Study the drawing (mm; zero at the part's minimum x, y, z) and answer. A direction names the side the tool comes from. Coordinates: 2 decimals unless noted, no trailing zeros. Loops run counter-clockwise (first coordinate to the right, second up) from the corner with the lowest first, then second, coordinate; pieces in that order, holes last. Notation, with made-up numbers: (-10.5, 16) -> (23.5, 16) arc R20 ccw to (23.5, 33) -> close; hole circle Ø1 at (78.5, -12). An arc over 180 degrees is marked (long way). Answer in a Markdown table with one row per item.
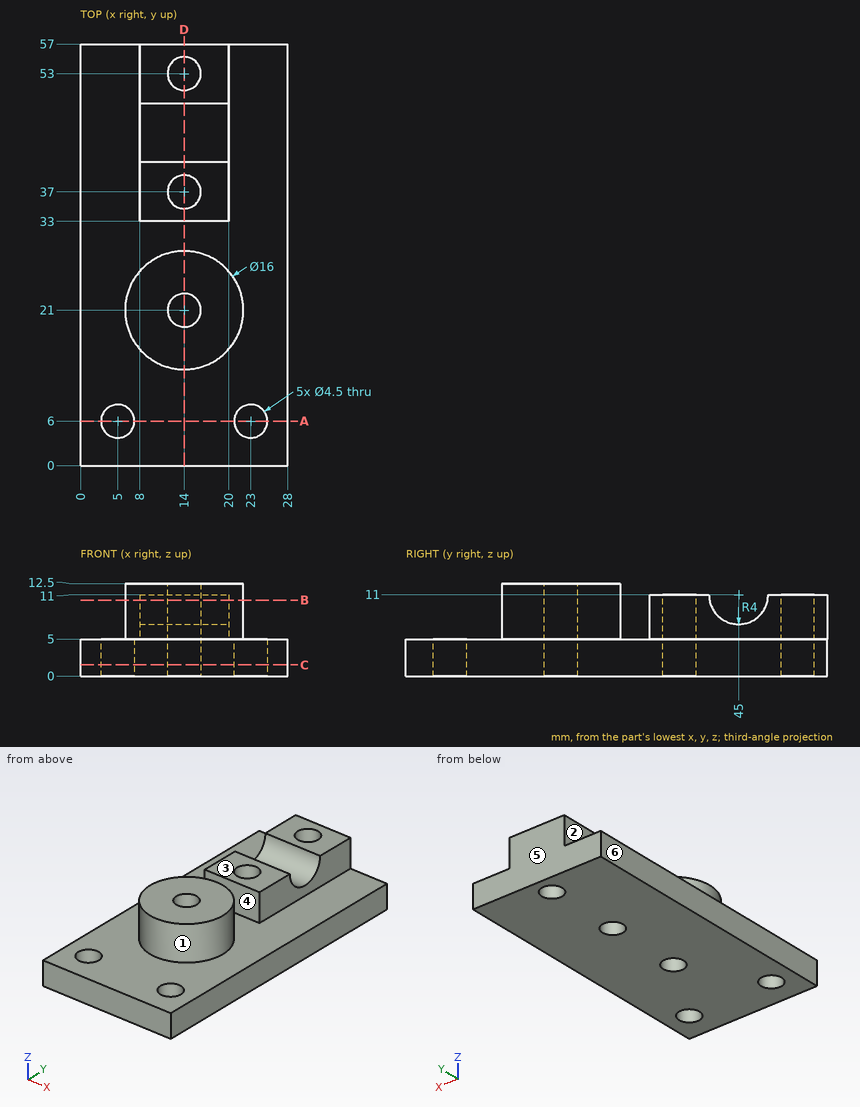
1. Given pin 1 Ø2.5 at (x, y) = (11.5, 38.5) entering from +Z; pin 2 Ø3 at (y, z) = (36, 8.5) entering from -X; pin 3 Ø1 at (y, z) = (46.5, 10.5) entering from -X; pin 4 Ø1.5 at (y, z) = (21.5, 7.5) entering from +X, each flat-ended and moving along its own axis, determine where each tip first touches the part or whether it passes through.
A:
| item | result |
|---|---|
| pin 1 | stops at z = 11 |
| pin 2 | stops at x = 8 |
| pin 3 | passes through |
| pin 4 | stops at x = 22 |
2. The mould has two halves that part along Y. Classify the marked faces 4, 5 and 6: pulls with the +Y half, pulls with the -Y half, needs draft (parallel to the pull), parting line crosses it, or undercut.
A:
| item | result |
|---|---|
| face 4 | undercut |
| face 5 | pulls with the +Y half |
| face 6 | needs draft |
3. A tool of negligible diameter and unlimited length cuts with its end or side. For the marked faces 1, 2 and 3, from which of +Z, -Z, +X, -X, +Y, -Y can it reach the whole face along a straight path? Write none if from no direction.
A:
| item | result |
|---|---|
| face 1 | +Z |
| face 2 | +Z, -X, +Y |
| face 3 | +Z, +X, -X, +Y |
4. A cutting plane is placed at A-A on y = 6. Give the vertices of the cut face in (x, z).
A:
| item | result |
|---|---|
| outline | (0, 0) -> (2.75, 0) -> (2.75, 5) -> (0, 5) -> close; (7.25, 0) -> (20.75, 0) -> (20.75, 5) -> (7.25, 5) -> close; (25.25, 0) -> (28, 0) -> (28, 5) -> (25.25, 5) -> close |
5. Find the intervals of material crossed by probe 1 along Y at (x, z) = (14, 8); probe 2 along Y at (x, z) = (16, 10.5); probe 3 along Y at (x, z) = (14, 6.5), in increasing order.
A:
| item | result |
|---|---|
| probe 1 | y = 13 to 18.75, 23.25 to 29, 33 to 34.75, 39.25 to 42.35, 47.65 to 50.75, 55.25 to 57 |
| probe 2 | y = 13.25 to 19.97, 22.03 to 28.75, 33 to 35.97, 38.03 to 41.03, 48.97 to 51.97, 54.03 to 57 |
| probe 3 | y = 13 to 18.75, 23.25 to 29, 33 to 34.75, 39.25 to 50.75, 55.25 to 57 |
6. A cutting plane is placed at C-C on z = 1.5. Give the vertices of the cut face in (x, y).
A:
| item | result |
|---|---|
| outline | (0, 0) -> (28, 0) -> (28, 57) -> (0, 57) -> close; hole circle Ø4.5 at (5, 6); hole circle Ø4.5 at (14, 21); hole circle Ø4.5 at (14, 37); hole circle Ø4.5 at (14, 53); hole circle Ø4.5 at (23, 6) |
7. A cutting plane is placed at D-D on x = 14. Give the vertices of the cut face in (y, z).
A:
| item | result |
|---|---|
| outline | (0, 0) -> (18.75, 0) -> (18.75, 12.5) -> (13, 12.5) -> (13, 5) -> (0, 5) -> close; (23.25, 0) -> (34.75, 0) -> (34.75, 11) -> (33, 11) -> (33, 5) -> (29, 5) -> (29, 12.5) -> (23.25, 12.5) -> close; (39.25, 0) -> (50.75, 0) -> (50.75, 11) -> (49, 11) arc R4 cw to (41, 11) -> (39.25, 11) -> close; (55.25, 0) -> (57, 0) -> (57, 11) -> (55.25, 11) -> close |
8. A cutting plane is placed at B-B on z = 10.25. Give the vertices of the cut face in (x, y).
A:
| item | result |
|---|---|
| outline | circle Ø16 at (14, 21); (8, 33) -> (20, 33) -> (20, 41.07) -> (8, 41.07) -> close; (8, 48.93) -> (20, 48.93) -> (20, 57) -> (8, 57) -> close; hole circle Ø4.5 at (14, 21); hole circle Ø4.5 at (14, 37); hole circle Ø4.5 at (14, 53) |
